Here's the drawing with two shaded views (mm, measured from the low corner). I have some questions. A direction names the side the tool comes from. Round coordinates to 2 decimals unless told otherwise and drop trailing zeros. Loops run counter-clockwise (first coordinate to the right, second up) from the corner with the lowest first, then second, coordinate; pieces in that order, holes last.
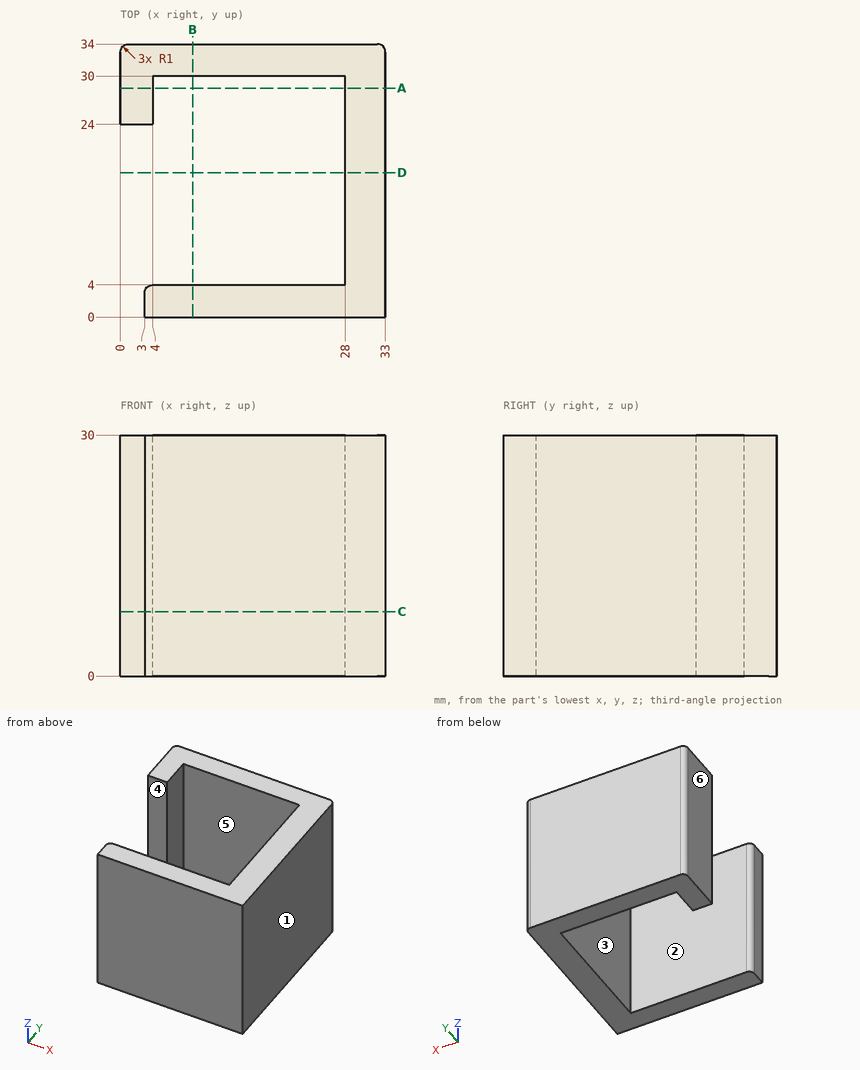
(1) If we section it at B-B, the plane x = 9: List the corners of the cut face in (y, z) for me.
Worked answers:
outline: (0, 0) - (4, 0) - (4, 30) - (0, 30) - close; (30, 0) - (34, 0) - (34, 30) - (30, 30) - close
(2) If I drill on line 1 (Y direction, x = 15, z = 8.5); line 2 (X direction, y = 28.5, z = 28); line 3 (X direction, y = 13, z = 20.5), over which ranges is the centre line in solid material (lowest first)?
Worked answers:
line 1: y = 0 to 4, 30 to 34
line 2: x = 0 to 4, 28 to 33
line 3: x = 28 to 33
(3) If we section it at A-A, the plane y = 28.5: List the corners of the cut face in (x, z) for me.
Worked answers:
outline: (0, 0) - (4, 0) - (4, 30) - (0, 30) - close; (28, 0) - (33, 0) - (33, 30) - (28, 30) - close
(4) For the marked faces 1, 2 and 3, which set-ups out of +Z, -Z, +X, -X, +Y, -Y let a thin tool reach every point of the face, with its end or its side?
Worked answers:
face 1: +Z, -Z, +X, +Y, -Y
face 2: +Z, -Z, -X
face 3: +Z, -Z
(5) If we mould it in two halves opening along X, with no side actions, what happens to the marked faces 4, 5 and 6? For each: released by +X, released by -X, zero draft, split by the parting line, or undercut.
Worked answers:
face 4: zero draft
face 5: undercut
face 6: released by -X
(6) If we section it at D-D, the plane y = 18: List the corners of the cut face in (x, z) for me, then the cut area to 3 significant figures.
Worked answers:
outline: (28, 0) - (33, 0) - (33, 30) - (28, 30) - close
area: 150 mm2
(7) If we section it at C-C, the plane z = 8: List the corners of the cut face in (x, y) for me, then the cut area to 3 significant figures.
Worked answers:
outline: (0, 24) - (4, 24) - (4, 30) - (28, 30) - (28, 4) - (4, 4) arc R1 ccw to (3, 3) - (3, 0) - (33, 0) - (33, 33) arc R1 ccw to (32, 34) - (1, 34) arc R1 ccw to (0, 33) - close
area: 405 mm2
(8) Will these pins go through, and if not, where does the flat tip stop? P1, Ø1.5, axis at y = 4, z = 18.5, coming from the -X side; P2, Ø3, axis at x = 12.5, y = 27, coming from the -Z side; P3, Ø8, axis at y = 15, z = 16.5, coming from the -X side.
Worked answers:
P1: stops at x = 3.03
P2: passes through
P3: stops at x = 28
